Drawing for the job (mm, zero at the part's lowest x, y, z). A direction names the side the tool comes from. Give positions to 0.01 mm unless a question says otherwise; leave off trailing zeros. Order: outer loops, then holes, each group sorted by start corner. A loop starts at its lowest first (then second) coordinate and runs counter-clockwise, first axis right, second up. Notation, with made-up numbers: (44.25, -8.5) -> (67.25, -8.5) arc R31 ccw to (67.25, 18.5) -> close; hole circle Ø6 at (61, 25). An arc over 180 degrees is marked (long way). Use one line per item in the form item = value. Start each with the question number.
1) Drop a flat-ended pin along its axis: P1, Ø8.5, axis at y = 18.5, z = 10, coming from the -X side. Give the stop position or say it passes through.
2) Mould opens along X. For the marked faces 1, 2 and 3 say: pulls with the +X half, pulls with the -X half, needs draft (parallel to the pull), parting line crosses it, or undercut.
3) Probe line 1 (Y direction, x = 8.7, z = 15); line 2 (X direction, y = 36, z = 24); line 3 (X direction, y = 6.5, z = 22.5). List the from-to ranges inside material, lowest first.
4) Cut at A-A, the plane z = 15. Give the cut face in (x, y).
5) Tool access for the marked faces 4, 5 and 6: list every direction of +Z, -Z, +X, -X, +Y, -Y with a clear straight run to the whole face (end or side of a thin tool).
6) Cut at C-C, the plane x = 24.5. Give the cut face in (y, z), and give its area (3 significant figures).
7) Cut at B-B, the plane y = 11. Give the cut face in (x, z), and give its area (3 significant figures).
8) Cut at D-D, the plane z = 3.5. Give the cut face in (x, y).
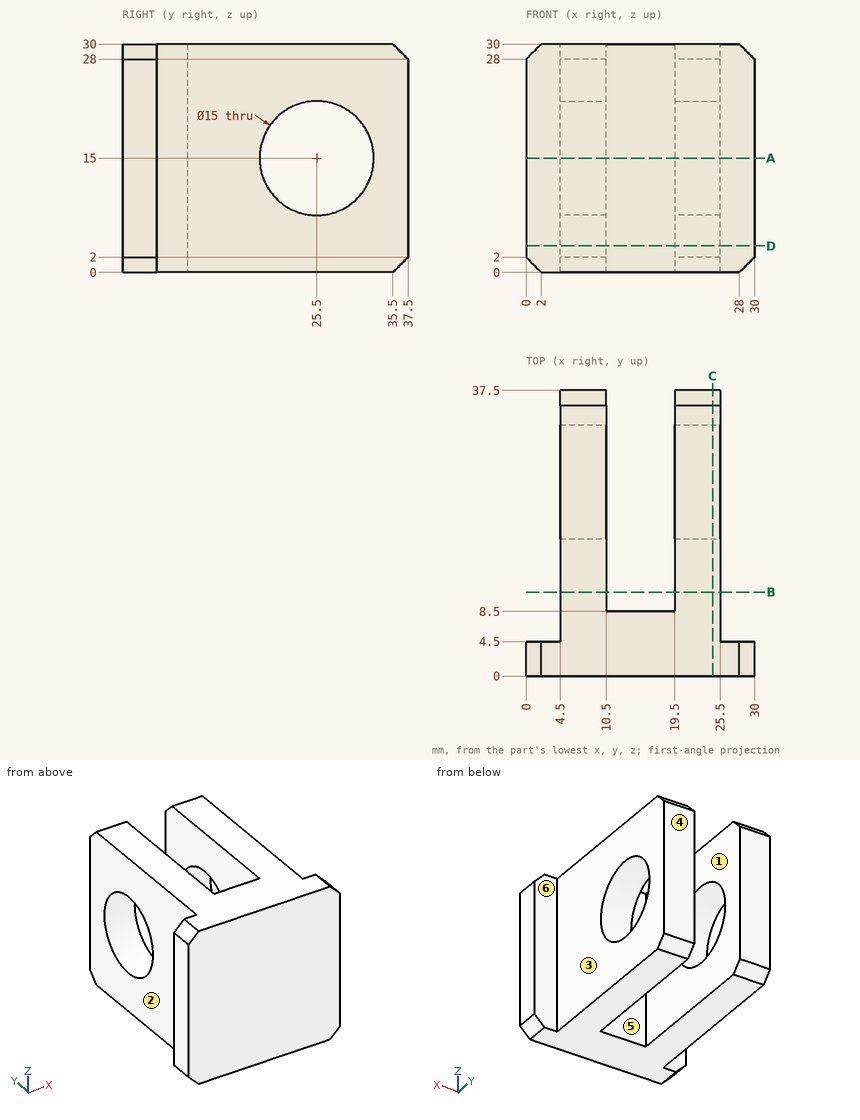
Result:
q1.P1 = 4.5
q2.face_1 = undercut
q2.face_2 = pulls with the -X half
q2.face_3 = pulls with the +X half
q3.line_1 = 0 to 18, 33 to 37.5
q3.line_2 = 4.5 to 10.5, 19.5 to 25.5
q3.line_3 = 4.5 to 25.5
q4.outline = (0, 0) -> (30, 0) -> (30, 4.5) -> (25.5, 4.5) -> (25.5, 18) -> (19.5, 18) -> (19.5, 8.5) -> (10.5, 8.5) -> (10.5, 18) -> (4.5, 18) -> (4.5, 4.5) -> (0, 4.5) -> close; (4.5, 33) -> (10.5, 33) -> (10.5, 37.5) -> (4.5, 37.5) -> close; (19.5, 33) -> (25.5, 33) -> (25.5, 37.5) -> (19.5, 37.5) -> close
q5.face_4 = +Z, -Z, +X, -X, +Y
q5.face_5 = +Z, -Z, +Y
q5.face_6 = +Z, -Z, +X, +Y
q6.outline = (0, 0) -> (35.5, 0) -> (37.5, 2) -> (37.5, 28) -> (35.5, 30) -> (0, 30) -> close; hole circle Ø15 at (25.5, 15)
q6.area = 944 mm²
q7.outline = (4.5, 0) -> (10.5, 0) -> (10.5, 30) -> (4.5, 30) -> close; (19.5, 0) -> (25.5, 0) -> (25.5, 30) -> (19.5, 30) -> close
q7.area = 360 mm²
q8.outline = (0, 0) -> (30, 0) -> (30, 4.5) -> (25.5, 4.5) -> (25.5, 37.5) -> (19.5, 37.5) -> (19.5, 8.5) -> (10.5, 8.5) -> (10.5, 37.5) -> (4.5, 37.5) -> (4.5, 4.5) -> (0, 4.5) -> close
